```python
from build123d import *

# Parameters (mm, degrees)
SKETCH1_W           = 5
SKETCH1_H           = 35
BOSS_EXTRUDE1_DEPTH = 5
SKETCH2_R           = 1
CUT_EXTRUDE1_DEPTH  = 19.874586088


with BuildPart() as part:
    # Sketch1 → Boss-Extrude1 (new body)
    with BuildSketch(Plane(origin=(0, 0, 0), x_dir=(1, 0, 0), z_dir=(0, 1, 0))):
        Rectangle(SKETCH1_W, SKETCH1_H)
    extrude(amount=BOSS_EXTRUDE1_DEPTH)

    # Sketch2 → Cut-Extrude1 (cut, through all)
    with BuildSketch(Plane(origin=(2.5, 0, 0), x_dir=(0, 0, -1), z_dir=(1, 0, 0))):
        with Locations((15, 2.5)):
            Circle(SKETCH2_R)
    cut_extrude1 = extrude(amount=-CUT_EXTRUDE1_DEPTH, mode=Mode.SUBTRACT)

    # Mirror1: Cut-Extrude1 across plane
    add(cut_extrude1.mirror(Plane.XY), mode=Mode.SUBTRACT)


solid = part.part
```
Geometry check sheet. Reference: the model listing, model coordinates, mm. Give positions to 0.01 mm unless a question says otherwise; leave off trailing zeros. Loops run counter-clockwise (first coordinate to the right, second up) from the corner with the lowest first, then second, coordinate; pieces in that order, holes last. Notation, with made-up numbers: M 27,78.25 L 76,78.25 A32 cw 76,116.25 Z; hole C 38.5,88.5 d5. An arc over 180 degrees is marked long. Write item = value, one per line. Start each with the question number.
1. Thickness scan on probe 1 along Y at (x, z) = (-0.9, -15); probe 2 along Z at (x, y) = (-0.15, 2.8). Record the ranges inside material, lowest first.
2. Section check A-A, the plane z = 15. Enter the section's corners in (x, y), plus the area to 3 significant figures.
3. Draft check along Z on faces 1 (the face through (0, 2, -17.5)), 2 (the face through (0.035, 2.8, -15.954)), 3 (the face through (2.5, 2, 0)). Enter one of: +Z half, -Z half, draft (parallel to the pull), parting line (faces both ways), or undercut.
4. Section check B-B, the plane y = 2.5. Enter the section's corners in (x, z), plus the area to 3 significant figures.
5. Section check C-C, the plane x = -0.65. Enter the section's corners in (y, z), plus the area to 3 significant figures.
Values follow:
q1.probe_1 = 0 to 1.5, 3.5 to 5
q1.probe_2 = -17.5 to -15.95, -14.05 to 14.05, 15.95 to 17.5
q2.outline = M -2.5,0 L 2.5,0 L 2.5,1.5 L -2.5,1.5 Z; M -2.5,3.5 L 2.5,3.5 L 2.5,5 L -2.5,5 Z
q2.area = 15.0 mm^2
q3.face_1 = -Z half
q3.face_2 = undercut
q3.face_3 = draft
q4.outline = M -2.5,-17.5 L 2.5,-17.5 L 2.5,-16 L -2.5,-16 Z; M -2.5,-14 L 2.5,-14 L 2.5,14 L -2.5,14 Z; M -2.5,16 L 2.5,16 L 2.5,17.5 L -2.5,17.5 Z
q4.area = 155 mm^2
q5.outline = M 0,-17.5 L 5,-17.5 L 5,17.5 L 0,17.5 Z; hole C 2.5,-15 d2; hole C 2.5,15 d2
q5.area = 169 mm^2
